```python
from build123d import *

# Parameters (mm, degrees)
SKETCH2_W           = 36
SKETCH2_H           = 36
BOSS_EXTRUDE1_DEPTH = 1.6
FILLET1_R           = 2.5
CUT_EXTRUDE1_REACH  = 27.506
SKETCH3_R           = 1.6


with BuildPart() as part:
    # Sketch2 → Boss-Extrude1 (new body)
    with BuildSketch(Plane.XY):
        Rectangle(SKETCH2_W, SKETCH2_H)
    extrude(amount=BOSS_EXTRUDE1_DEPTH)

    # Fillet1
    fillet1_edges = [part.edges().sort_by_distance(p)[0] for p in [
        (-18, 18, 0.8),
        (18, 18, 0.8),
        (18, -18, 0.8),
        (-18, -18, 0.8),
    ]]
    fillet(fillet1_edges, radius=FILLET1_R)

    # Sketch3 → Cut-Extrude1 (cut, up to next)
    with BuildSketch(Plane.XY.offset(1.6), mode=Mode.PRIVATE) as cut_extrude1_sk1:
        with Locations((-15.5, -15.5)):
            Circle(SKETCH3_R)
    cut_extrude1_tool1 = extrude(cut_extrude1_sk1.sketch, amount=-CUT_EXTRUDE1_REACH, mode=Mode.PRIVATE) & part.part
    # Sketch3 → Cut-Extrude1 (cut, up to next)
    with BuildSketch(Plane.XY.offset(1.6), mode=Mode.PRIVATE) as cut_extrude1_sk2:
        with Locations((-15.5, 15.5)):
            Circle(SKETCH3_R)
    cut_extrude1_tool2 = extrude(cut_extrude1_sk2.sketch, amount=-CUT_EXTRUDE1_REACH, mode=Mode.PRIVATE) & part.part
    # Sketch3 → Cut-Extrude1 (cut, up to next)
    with BuildSketch(Plane.XY.offset(1.6), mode=Mode.PRIVATE) as cut_extrude1_sk3:
        with Locations((15.48525874, 15.5)):
            Circle(SKETCH3_R)
    cut_extrude1_tool3 = extrude(cut_extrude1_sk3.sketch, amount=-CUT_EXTRUDE1_REACH, mode=Mode.PRIVATE) & part.part
    # Sketch3 → Cut-Extrude1 (cut, up to next)
    with BuildSketch(Plane.XY.offset(1.6), mode=Mode.PRIVATE) as cut_extrude1_sk4:
        with Locations((15.5, -15.5)):
            Circle(SKETCH3_R)
    cut_extrude1_tool4 = extrude(cut_extrude1_sk4.sketch, amount=-CUT_EXTRUDE1_REACH, mode=Mode.PRIVATE) & part.part
    add(cut_extrude1_tool1.solids().sort_by_distance((-15.5, -15.5, 1.6))[0], mode=Mode.SUBTRACT)
    add(cut_extrude1_tool2.solids().sort_by_distance((-15.5, 15.5, 1.6))[0], mode=Mode.SUBTRACT)
    add(cut_extrude1_tool3.solids().sort_by_distance((15.485259, 15.5, 1.6))[0], mode=Mode.SUBTRACT)
    add(cut_extrude1_tool4.solids().sort_by_distance((15.5, -15.5, 1.6))[0], mode=Mode.SUBTRACT)


solid = part.part
```
Check sheet for the modelled part. Datum: model origin and axes. Units: mm. Round coordinates to 2 decimals unless told otherwise and drop trailing zeros. Loops run counter-clockwise (first coordinate to the right, second up) from the corner with the lowest first, then second, coordinate; pieces in that order, holes last. Notation, with made-up numbers: (-15.5, 30) - (16.5, 30) arc R15 cw to (16.5, 54) - close; hole circle Ø4 at (54.25, 57.25). An arc over 180 degrees is marked (long way). Write item = value, one per line. Start each with the question number.
Q1. Section check B-B (x = -14.5). Record the boundary of the cut face in (y, z).
Q2. Section check A-A (z = 1.1). Record the boundary of the cut face in (x, y).
Q3. Thickness scan on L1, parallel to Y at x = -15.5, z = 0.4; L2, parallel to Y at x = -15, z = 0.9; L3, parallel to X at y = -16, z = 0.5. Record the ranges inside material, lowest first.
Q4. Release check for a two-part mould opening along Y. For faces 1 (the face through (0, 0, 0)), 2 (the face through (17.248, -17.287, 0.811)), 3 (the face through (0, 18, 1)), 4 (the face through (13.9, -15.43, 0.81)) record: pulls with the +Y half, pulls with the -Y half, needs draft (parallel to the pull), parting line crosses it, or undercut.
Derived:
q1.outline = (-18, 0) - (-16.75, 0) - (-16.75, 1.6) - (-18, 1.6) - close; (-14.25, 0) - (14.25, 0) - (14.25, 1.6) - (-14.25, 1.6) - close; (16.75, 0) - (18, 0) - (18, 1.6) - (16.75, 1.6) - close
q2.outline = (-18, -15.5) arc R2.5 ccw to (-15.5, -18) - (15.5, -18) arc R2.5 ccw to (18, -15.5) - (18, 15.5) arc R2.5 ccw to (15.5, 18) - (-15.5, 18) arc R2.5 ccw to (-18, 15.5) - close; hole circle Ø3.2 at (-15.5, -15.5); hole circle Ø3.2 at (-15.5, 15.5); hole circle Ø3.2 at (15.49, 15.5); hole circle Ø3.2 at (15.5, -15.5)
q3.L1 = -18 to -17.1, -13.9 to 13.9, 17.1 to 18
q3.L2 = -18 to -17.02, -13.98 to 13.98, 17.02 to 18
q3.L3 = -17.95 to -17.02, -13.98 to 13.98, 17.02 to 17.95
q4.face_1 = needs draft
q4.face_2 = pulls with the -Y half
q4.face_3 = pulls with the +Y half
q4.face_4 = undercut
